Check sheet for the modelled part. Datum: model origin and axes. Units: mm. Face numbers are marked on the shaded views. Give positions to 0.01 mm unless a question says otherwise; leave off trailing zeros. Order: outer loops, then holes, each group sorted by start corner. A loop starts at its lowest first (then second) coordinate and runs counter-clockwise, first axis right, second up.
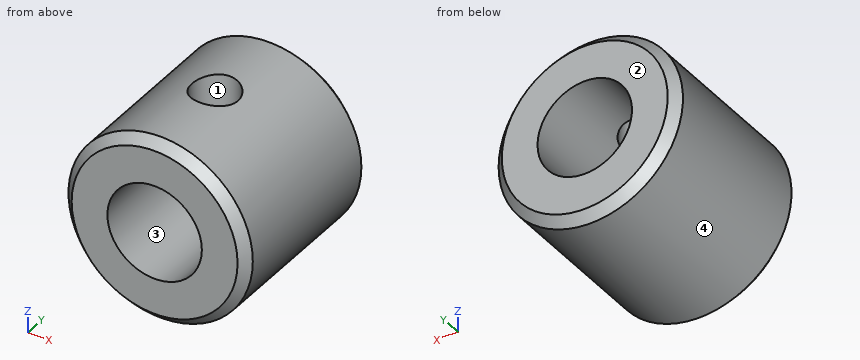
from build123d import *

# Parameters (mm, degrees)
F0_R     = 10
F0_R_2   = 5.125
F1_DEPTH = 20
F3_D     = 5
F3_DEPTH = 10.001
F4_SIZE  = 1


with BuildPart() as f1:
    # F0 (on Front) → F1 (new body)
    with BuildSketch(Plane.XZ):
        Circle(F0_R)
        Circle(F0_R_2, mode=Mode.SUBTRACT)
    extrude(amount=F1_DEPTH)

    # F3 (through all, one way)
    with BuildSketch(Plane(origin=(0, 0, 0), x_dir=(1, 0, 0), z_dir=(0, 0, -1))):
        with Locations((0, 10)):
            Circle(F3_D / 2)
    extrude(amount=-F3_DEPTH, mode=Mode.SUBTRACT)

    # F4
    f4_edges = [f1.edges().sort_by_distance(p)[0] for p in [
        (-10, -20, 0),
        (-10, 0, 0),
    ]]
    chamfer(f4_edges, length=F4_SIZE)


solid = f1.part
1) Material ranges on L1, parallel to Y at x = 0, z = 6.2; L2, parallel to X at y = -10, z = 7.05; L3, parallel to X at y = -10, z = 8.4, recorded low to high.
Recorded:
L1: y = -20 to -12.5, -7.5 to 0
L2: x = -7.09 to -2.5, 2.5 to 7.09
L3: x = -5.43 to -2.5, 2.5 to 5.43
2) Section check B-B, the plane z = 0. Record the cut outline in (x, y) (3 decimals), then the cut area to 3 significant figures.
Recorded:
outline: (-10, -19) - (-9, -20) - (-5.125, -20) - (-5.125, 0) - (-9, 0) - (-10, -1) - close; (5.125, -20) - (9, -20) - (10, -19) - (10, -1) - (9, 0) - (5.125, 0) - close
area: 193 mm2
3) Depth check by flat-ended pin: pin 1 Ø3 at (y, z) = (-12.5, -6) entering from +X; pin 2 Ø1.5 at (x, y) = (-4, -16.5) entering from -Z. Enter the tip coordinate at first touch or a pass-through.
Recorded:
pin 1: stops at x = 8.93
pin 2: stops at z = -9.46
4) Draft check along X on the marked faces 1, 2, 3 and 4. Enter one of: +X half, -X half, draft (parallel to the pull), parting line (faces both ways), or undercut.
Recorded:
face 1: undercut
face 2: draft
face 3: undercut
face 4: parting line
5) Section check C-C, the plane y = -17. Record the cut outline in (x, z) (3 decimals), then the cut area to 3 significant figures.
Recorded:
outline: circle Ø20 at (0, 0); hole circle Ø10.25 at (0, 0)
area: 232 mm2
6) Section check A-A, the plane x = 0. Record the cut outline in (y, z) (3 decimals), then the cut area to 3 significant figures.
Recorded:
outline: (-20, -9) - (-19, -10) - (-1, -10) - (0, -9) - (0, -5.125) - (-20, -5.125) - close; (-20, 5.125) - (-12.5, 5.125) - (-12.5, 10) - (-19, 10) - (-20, 9) - close; (-7.5, 5.125) - (0, 5.125) - (0, 9) - (-1, 10) - (-7.5, 10) - close
area: 169 mm2
7) Section check D-D, the plane y = -10. Record the cut outline in (x, z) (3 decimals), then the cut area to 3 significant figures.
Recorded:
outline: (-2.5, 4.474) - (-2.5, 9.682) arc R10 ccw (long way) to (2.5, 9.682) - (2.5, 4.474) arc R5.125 cw (long way) to start
area: 207 mm2
